Build history of the part. All positions in model axes, mm. Face numbers are marked on the shaded views. A direction names the side the tool comes from. Round coordinates to 2 decimals unless told otherwise and drop trailing zeros. Loops run counter-clockwise (first coordinate to the right, second up) from the corner with the lowest first, then second, coordinate; pieces in that order, holes last.
from build123d import *
from build123d.topology import SkipClean

# Parameters (mm, degrees)
SKIZZE1_R                       = 50
AUFSATZ_LINEAR_AUSTRAGEN1_DEPTH = 3
SKIZZE7_R                       = 5.030567549
SKIZZE7_R_2                     = 5
AUFSATZ_LINEAR_AUSTRAGEN4_DEPTH = 20
AUFSATZ_LINEAR_START            = -2
SKIZZE8_R                       = 45
AUFSATZ_LINEAR_AUSTRAGEN5_DEPTH = 2
SKIZZE9_R                       = 2.5
SCHNITT_LINEAR_AUSTRAGEN1_DEPTH = 2
SKIZZE10_R                      = 1.9
SCHNITT_LINEAR_AUSTRAGEN2_DEPTH = 18


with BuildPart() as part:
    # Skizze1 → Aufsatz-Linear austragen1 (new body)
    with BuildSketch(Plane(origin=(0, 0, 0), x_dir=(1, 0, 0), z_dir=(0, 1, 0))):
        with Locations(Location((0, 0, 0), (0, 0, 270))):
            Circle(SKIZZE1_R)
        with BuildLine():
            ThreePointArc((-4.992277988, 44.722222222), (0, 40), (4.992277988, 44.722222222))
            ThreePointArc((4.992277988, 44.722222222), (38.97114317, 22.5), (41.226719552, -18.037671551))
            ThreePointArc((41.226719552, -18.037671551), (34.641016151, -20), (36.234441564, -26.684550671))
            ThreePointArc((36.234441564, -26.684550671), (-0.858918242, -44.991802136), (-37.226514275, -25.282140632))
            ThreePointArc((-37.226514275, -25.282140632), (-35.37911937, -18.663277112), (-41.88512765, -16.451020689))
            ThreePointArc((-41.88512765, -16.451020689), (-38.534584491, 23.239746085), (-4.992277988, 44.722222222))
        make_face(mode=Mode.SUBTRACT)
    extrude(amount=AUFSATZ_LINEAR_AUSTRAGEN1_DEPTH)

    # Skizze4 → Rotation1 (revolve)
    with BuildSketch(Plane.XY, mode=Mode.PRIVATE) as rotation1_sk:
        Polygon((-45, 20), (-50, 3), (-45, 3), (-40, 20), align=None)
    revolve(rotation1_sk.sketch.rotate(Axis((0, 0, 0), (0, 1, 0)), 270), axis=Axis((0, 0, 0), (0, 1, 0)))

    # Skizze7 → Aufsatz-Linear austragen4 (add)
    with SkipClean():  # the faces are left unmerged after this step: merging them gives an invalid solid
        with BuildSketch(Plane.XZ):
            with Locations((-39.801509292, 20.996186751)):
                Circle(SKIZZE7_R)
            with Locations((0, -45)):
                Circle(SKIZZE7_R_2)
            with Locations((38.97114317, 22.5)):
                Circle(SKIZZE7_R_2)
        extrude(amount=-AUFSATZ_LINEAR_AUSTRAGEN4_DEPTH)

    # Skizze8 → Aufsatz-Linear austragen5 (add)
    with BuildSketch(Plane(origin=(0, 20, 0), x_dir=(1, 0, 0), z_dir=(0, 1, 0)).offset(AUFSATZ_LINEAR_START)):
        Circle(SKIZZE8_R)
    extrude(amount=AUFSATZ_LINEAR_AUSTRAGEN5_DEPTH)

    # Skizze9 → Schnitt-Linear austragen1 (cut)
    with BuildSketch(Plane(origin=(0, 20, 0), x_dir=(1, 0, 0), z_dir=(0, 1, 0))):
        with BuildLine():
            ThreePointArc((-1.885847319, 20.741185347), (-5.455813521, 18.385669713), (-6.988967253, 14.392857143))
            ThreePointArc((-6.988967253, 14.392857143), (0, -16), (6.988967253, 14.392857143))
            ThreePointArc((6.988967253, 14.392857143), (4.072563813, 19.693349101), (-1.885847319, 20.741185347))
        make_face()
        with Locations(Location((0, 28, 0), (0, 0, 270))):
            Circle(SKIZZE9_R)
    extrude(amount=-SCHNITT_LINEAR_AUSTRAGEN1_DEPTH, mode=Mode.SUBTRACT)

    # Skizze10 → Schnitt-Linear austragen2 (cut)
    with BuildSketch(Plane.XZ):
        with Locations(Location((-39.801509292, 20.996186751, 0), (0, 0, 270))):
            Circle(SKIZZE10_R)
        with Locations(Location((38.97114317, 22.5, 0), (0, 0, 270))):
            Circle(SKIZZE10_R)
        with Locations(Location((0, -45, 0), (0, 0, 270))):
            Circle(SKIZZE10_R)
    extrude(amount=-SCHNITT_LINEAR_AUSTRAGEN2_DEPTH, mode=Mode.SUBTRACT)


solid = part.part
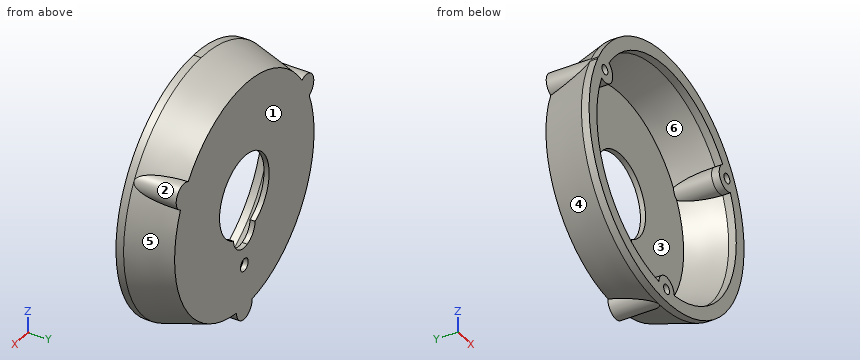
(1) Pin check, flat tips, straight feed: P1, Ø1, axis at y = 15, z = -26, coming from the +X side; P2, Ø4, axis at x = -4, y = 8, coming from the +Z side; P3, Ø12, axis at x = -14, y = 13, coming from the -Z side; P4, Ø4, axis at x = 0, z = -28, coming from the -Y side. Stop position of each tip, or through.
Responses:
P1: stops at x = 38.89
P2: stops at z = 48.97
P3: stops at z = -47.34
P4: passes through
(2) Which spindle directions (+Z, -Z, +X, -X, +Y, -Y) get a long thin tool onto all of the face, cutting with end or side? Do the marked faces 1, 2 and 3. Say none if no direction does.
Responses:
face 1: +Z, -Z, +X, -X, +Y
face 2: +Y
face 3: -Y
(3) Slice it at C-C on y = 7. List the corners of the cut face in (x, z), plus the area to 3 significant figures.
Responses:
outline: (-44.67, 19.71) arc R48.82 ccw to (-3.35, -48.71) arc R5 ccw to (3.35, -48.71) arc R48.82 ccw to (43.86, 21.45) arc R5 ccw to (40.51, 27.26) arc R48.82 ccw to (-41.49, 25.73) arc R5.03 ccw to start; hole circle Ø3.8 at (-39.8, 21); hole (-40.77, 16.06) arc R43.82 ccw to (-4.79, -43.56) arc R5 cw to (4.79, -43.56) arc R43.82 ccw to (40.12, 17.63) arc R5 cw to (35.33, 25.93) arc R43.82 ccw to (-36.28, 24.59) arc R5.03 cw to start; hole circle Ø3.8 at (0, -45); hole circle Ø3.8 at (38.97, 22.5)
area: 1,520 mm2
(4) Slice it at A-A on z = 0. List the corners of the cut face in (x, y).
Responses:
outline: (-50, 0) - (-45, 0) - (-45, 3) - (-40.59, 18) - (-16, 18) - (-16, 20) - (-45, 20) - (-50, 3) - close; (16, 18) - (40.59, 18) - (45, 3) - (45, 0) - (50, 0) - (50, 3) - (45, 20) - (16, 20) - close
(5) Probe line 1 (Z direction, x = 1, y = 6.5); line 2 (Z direction, x = -38.5, y = 8); line 3 (Y direction, x = 30, z = -12). List the from-to ranges inside material, lowest first.
Responses:
line 1: z = -49.9 to -46.62, -43.38 to -40.1, 43.96 to 48.96
line 2: z = -29.54 to -20.31, 16.14 to 19.61, 22.38 to 29.54
line 3: y = 18 to 20
(6) Pull direction X, two halves, no side cores. Call the marked faces 4, 5 and 6: +X half, -X half, draft (parallel to the pull), parting line (faces both ways), or undercut.
Responses:
face 4: -X half
face 5: +X half
face 6: undercut
(7) Slice it at B-B on y = 12.75. List the corners of the cut face in (x, z).
Responses:
outline: (-43.66, 17.76) arc R47.13 ccw to (-4.62, -46.91) arc R5 ccw to (4.62, -46.91) arc R47.13 ccw to (42.93, 19.45) arc R5 ccw to (38.31, 27.46) arc R47.13 ccw to (-39.31, 26) arc R5.03 ccw to start; hole circle Ø3.8 at (-39.8, 21); hole (-38.96, 16.04) arc R42.13 ccw to (-3.96, -41.95) arc R5 cw to (3.96, -41.95) arc R42.13 ccw to (38.31, 17.54) arc R5 cw to (34.35, 24.4) arc R42.13 ccw to (-35.23, 23.1) arc R5.03 cw to start; hole circle Ø3.8 at (0, -45); hole circle Ø3.8 at (38.97, 22.5)
